Source: CAD feature listing. Evaluate the final solid. Frame: model axes, mm. Round coordinates to 2 decimals unless told otherwise and drop trailing zeros. Write each loop counter-clockwise with the first axis right and the second up, starting at its lowest first coordinate (ties: lowest second). Pieces come first, ordered by that corner, then holes.
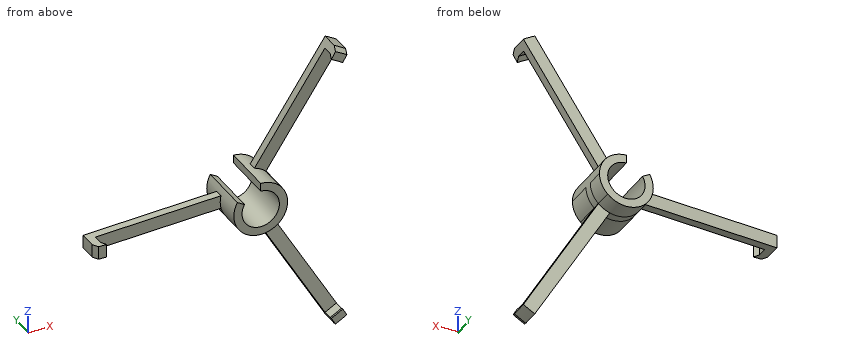
from build123d import *
from build123d import SkipClean  # not in build123d's __all__

# Parameters (mm, degrees)
F3_DEPTH = 25.4


with BuildPart() as f1:
    # F0 (on Top) → F1 (revolve)
    with BuildSketch(Plane.XY):
        Polygon((63.7286, -3.81), (63.7286, 2.9399013527), (10.3759, 7.0484601322), (10.3759, 13.97), (7.2009, 13.97), (7.2009, -6.35), (10.3759, -6.35), (10.3759, 3.8640599232), (60.5536, 0), (60.5536, -3.81), (59.2836, -6.0097045256), (62.4586, -6.0097045256), align=None)
    revolve(axis=Axis((0, -13.2026916835, 0), (0, -1, 0)))

    # F2 (on face) → F3 (cut)
    with BuildSketch(Plane(origin=(0, 13.97, 0), x_dir=(-1, 0, 0), z_dir=(0, 1, 0))):
        with BuildLine():
            Line((111.0251099892, -2.54), (10.0602038155, -2.54))
            ThreePointArc((10.0602038155, -2.54), (5.18795, -8.9857929871), (-2.8303973822, -9.9823920715))
            Line((-2.8303973822, -9.9823920715), (-53.312850469, -97.4205657086))
            ThreePointArc((-53.312850469, -97.4205657086), (40.7588842751, -70.5964584242), (111.0251099892, -2.54))
        make_face()
        with BuildLine():
            Line((10.0602038155, 2.54), (111.0251099892, 2.54))
            ThreePointArc((111.0251099892, 2.54), (40.7588842751, 70.5964584242), (-53.312850469, 97.4205657086))
            Line((-53.312850469, 97.4205657086), (-2.8303973822, 9.9823920715))
            ThreePointArc((-2.8303973822, 9.9823920715), (-1.4288105045, 10.2770521723), (0, 10.3759))
            Line((0, 10.3759), (0, 0))
            Line((0, 0), (8.9857929871, 5.18795))
            ThreePointArc((8.9857929871, 5.18795), (9.6145935095, 3.9011398921), (10.0602038155, 2.54))
        make_face()
        with BuildLine():
            Line((-7.2298064334, 7.4423920715), (-57.7122595202, 94.8805657086))
            ThreePointArc((-57.7122595202, 94.8805657086), (-81.5177685501, 0), (-57.7122595202, -94.8805657086))
            Line((-57.7122595202, -94.8805657086), (-7.2298064334, -7.4423920715))
            ThreePointArc((-7.2298064334, -7.4423920715), (-10.3759, 0), (-7.2298064334, 7.4423920715))
        make_face()
    with SkipClean():  # cleaning this boolean's faces spoils the solid; the shape is the same uncleaned
        extrude(amount=-F3_DEPTH, mode=Mode.SUBTRACT)


solid = f1.part
1) Section query B-B on y = 9.25. Return the cut outline in (x, z), then the cut area to 3 significant figures.
Taken from the geometry:
outline: (-8.99, 5.19) arc R10.38 ccw (long way) to (0, 10.38) - (0, 7.2) arc R7.2 cw (long way) to (-6.24, 3.6) - close
area: 146 mm2
2) Section query A-A on y = -2. Return the cut outline in (x, z).
Taken from the geometry:
outline: (-63.68, -2.54) - (-60.5, -2.54) arc R60.55 cw to (-60.5, 2.54) - (-63.68, 2.54) arc R63.73 ccw to start; (-8.99, 5.19) arc R10.38 ccw (long way) to (0, 10.38) - (0, 7.2) arc R7.2 cw (long way) to (-6.24, 3.6) - close; (28.05, -53.66) - (29.64, -56.42) arc R63.73 ccw to (34.04, -53.88) - (32.45, -51.12) arc R60.55 cw to start; (28.05, 53.66) arc R60.55 cw to (32.45, 51.12) - (34.04, 53.88) arc R63.73 ccw to (29.64, 56.42) - close
3) Material intervals for line 1 (X direction, y = 7.25, z = 0); line 2 (Z direction, x = 3.5, y = 6.75); line 3 (Z direction, x = -45, y = 2.75), sorted ascending.
Taken from the geometry:
line 1: x = -10.38 to -7.2, 7.2 to 10.38
line 2: z = -11.14 to -6.29, 6.29 to 11.14
line 3: z = -2.54 to 2.54
4) Contact query for flat-ended pins moving along their axis: P1, Ø12, axis at y = 4, z = 18, coming from the -X side; P2, Ø3.5, axis at y = 7.5, z = 8, coming from the -X side; P3, Ø1, axis at x = -45, z = -1, coming from the -Y side; P4, Ø8, axis at x = 0, z = 18, coming from the +Y side. Output: stop coordinate, or through.
Taken from the geometry:
P1: stops at x = 4
P2: stops at x = 0
P3: stops at y = 1.16
P4: passes through
